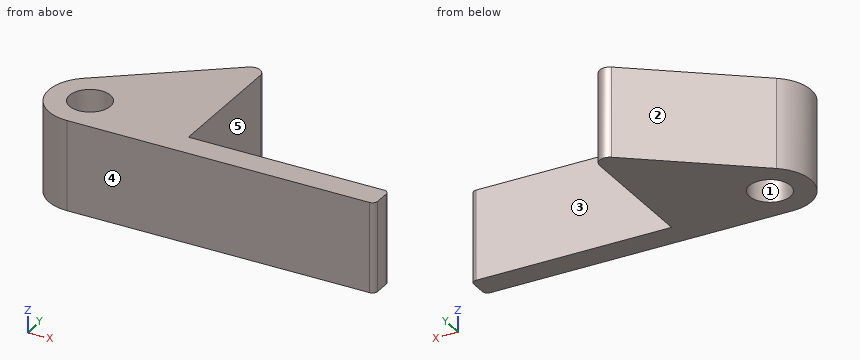
```python
from build123d import *

# Parameters (mm, degrees)
ESQUISSE1_R        = 8
ESQUISSE1_R_2      = 4
BOSS_EXTRU_2_DEPTH = 17.5
CONG_1_R           = 2
CONG_2_R           = 1


with BuildPart() as part:
    # Esquisse1 → Boss.-Extru.2 (new body)
    # profile 1 of 2: a face of its own
    with BuildSketch(Plane.XY):
        with BuildLine():
            Line((20.866963315, 26), (-4.855214383, 6.358214631))
            ThreePointArc((-4.855214383, 6.358214631), (3.546708681, 7.17083381), (8, 0))
            ThreePointArc((8, 0), (5.656854249, -5.656854249), (0, -8))
            Line((0, -8), (60, -8))
            Line((60, -8), (60, -3))
            Line((60, -3), (20.866963315, -3))
            Line((20.866963315, -3), (20.866963315, 26))
        make_face()
    # profile 2 of 2: a face of its own
    with BuildSketch(Plane.XY):
        Circle(ESQUISSE1_R)
        Circle(ESQUISSE1_R_2, mode=Mode.SUBTRACT)
    extrude(amount=-BOSS_EXTRU_2_DEPTH)

    # Congé1
    cong_1_edges = [part.edges().sort_by_distance(p)[0] for p in [
        (20.866963315, 26, -8.75),
    ]]
    fillet(cong_1_edges, radius=CONG_1_R)

    # Congé2
    cong_2_edges = [part.edges().sort_by_distance(p)[0] for p in [
        (60, -3, -8.75),
        (60, -8, -8.75),
    ]]
    fillet(cong_2_edges, radius=CONG_2_R)


solid = part.part
```
Geometry: final body of the model. Coordinates: model frame, mm. Face numbers are marked on the shaded views. A direction names the side the tool comes from. Coordinates: 2 decimals unless noted, no trailing zeros. Order: outer loops, then holes, each group sorted by start corner. A loop starts at its lowest first (then second) coordinate and runs counter-clockwise, first axis right, second up. Notation, with made-up numbers: (33, -24.5) -> (83, -24.5) arc R16 cw to (83, -15.5) -> close; hole circle Ø4 at (46.25, -14). An arc over 180 degrees is marked (long way). Use CSV: the item, a comma, the result in double quotes.
1) Access query for the marked faces 4 and 5. Directions: +Z, -Z, +X, -X, +Y, -Y. A direction counts if a zero-diameter tool reaches every point of the face in a straight line with its end or side. Return the directions, or none.
Findings:
face 4,"+Z, -Z, +X, -X, -Y"
face 5,"+Z, -Z, +X, +Y"
2) Section B-B on z = -14.75. Output: boundary loops of the cut face in (x, y), then the cut area to 3 significant figures.
Findings:
outline,"(-4.86, 6.36) arc R8 ccw to (0, -8) -> (59, -8) arc R1 ccw to (60, -7) -> (60, -4) arc R1 ccw to (59, -3) -> (20.87, -3) -> (20.87, 21.96) arc R2 ccw to (17.65, 23.55) -> close; hole circle Ø8 at (0, 0)"
area,"789 mm^2"
3) Section D-D on y = 17. Output: boundary loops of the cut face in (x, z), then the cut area to 3 significant figures.
Findings:
outline,"(9.08, -17.5) -> (20.87, -17.5) -> (20.87, 0) -> (9.08, 0) -> close"
area,"206 mm^2"
4) Pin query (flat end, axial travel): pin 1 Ø1.5 at (y, z) = (12, -13) entering from -X; pin 2 Ø1 at (y, z) = (5.5, -4) entering from +X; pin 3 Ø5 at (x, z) = (45, -6.5) entering from +Y. Return the tip coordinate at first contact, or that it passes through.
Findings:
pin 1,"stops at x = 1.55"
pin 2,"stops at x = 20.87"
pin 3,"stops at y = -3"
5) Section C-C on x = 16. Output: boundary loops of the cut face in (y, z).
Findings:
outline,"(-8, -17.5) -> (22.28, -17.5) -> (22.28, 0) -> (-8, 0) -> close"
6) Mould query, pull axis X, two halves, no side actions, for the marked faces 1, 2 and 3. Classes: +X half, -X half, draft (parallel to the pull), parting line (faces both ways), or undercut.
Findings:
face 1,"undercut"
face 2,"-X half"
face 3,"draft"
7) Line query: line 1 (Y direction, x = 34.5, z = -6.25); line 2 (X direction, y = 0.5, z = -1.25); line 3 (Y direction, x = 3.5, z = -2.5). Output: solid intervals per line, ascending.
Findings:
line 1,"y = -8 to -3"
line 2,"x = -7.98 to -3.97, 3.97 to 20.87"
line 3,"y = -8 to -1.94, 1.94 to 12.74"
8) Section A-A on y = 0. Output: boundary loops of the cut face in (x, z), then the cut area to 3 significant figures.
Findings:
outline,"(-8, -17.5) -> (-4, -17.5) -> (-4, 0) -> (-8, 0) -> close; (4, -17.5) -> (20.87, -17.5) -> (20.87, 0) -> (4, 0) -> close"
area,"365 mm^2"
